The model under review builds one solid part; all positions refer to its coordinate system, in mm. A direction names the side the tool comes from. Coordinates: 2 decimals unless noted, no trailing zeros. Loops run counter-clockwise (first coordinate to the right, second up) from the corner with the lowest first, then second, coordinate; pieces in that order, holes last. Notation, with made-up numbers: (15.25, 17) - (56.25, 17) arc R19 ccw to (56.25, 52) - close; hole circle Ø11 at (1, 8). An arc over 180 degrees is marked (long way). One line per item, written item: value. Start each with the question number.
1. For faces 1 (the face through (7, -1.83, 10)), 2 (the face through (3, 4.99, -5)), list the 3-axis set-ups (+Z, -Z, +X, -X, +Y, -Y) from which the entire face can be reached by the end or side of a thin tool; tool diameter is ignored.
2. We need section A-A, the plane z = 0. Give the boundary of the cut face in (x, y).
3. Mouldability with a two-part tool opening along Y and no side actions: class faces 3 (the face through (11.74, 2.78, 2.61)), 4 (the face through (11.797, 1.658, -6.136)), 5 (the face through (-0.2, 6.26, 5.3)) as +Y half, -Y half, draft (parallel to the pull), parting line (faces both ways), or undercut.
4. Insertion check: P1, Ø4, axis at x = 1.5, y = 2, coming from the +Z side; P2, Ø1.5, axis at x = -4, y = 2, coming from the -Z side; P3, Ø14.5, axis at x = 0, z = 0, coming from the -Y side. Each pin has a flat end and moves straight along its axis. Give the tip position at first contact, or say it passes through.
5. We need section C-C, the plane y = 2.75. Give the boundary of the cut face in (x, z), then the cut area to 3 significant figures.
6. We need section B-B, the plane x = 0. Give the boundary of the cut face in (y, z), then the cut area to 3 significant figures.
7. To check wall thickness, follow line 1 (X direction, y = 3.5, z = 0); line 2 (Z direction, x = -2.75, y = 0); line 3 (Y direction, x = 1.5, z = -8.75). State the ranges of each line that lie inside material, in increasing order.
8. We need section D-D, the plane y = -1. Give the boundary of the cut face in (x, z), then the cut area to 3 significant figures.
from build123d import *


with BuildPart() as part:
    # Sketch1 → Revolve1 (revolve)
    with BuildSketch(Plane.XY, mode=Mode.PRIVATE) as revolve1_sk:
        with BuildLine():
            Line((12.0269, 0.508129433), (12.0269, 4.990057463))
            Line((12.0269, 4.990057463), (5.207, 4.990057463))
            Line((5.207, 4.990057463), (5.08, 6.260057463))
            Line((5.08, 6.260057463), (12.2809, 6.260057463))
            ThreePointArc((12.2809, 6.260057463), (12.99932049, 5.962477952), (13.2969, 5.244057463))
            Line((13.2969, 5.244057463), (13.2969, -1.829842537))
            Line((13.2969, -1.829842537), (12.0269, -1.829842537))
            ThreePointArc((12.0269, -1.829842537), (11.330182262, -0.940102098), (11.802382058, 0.086582375))
            ThreePointArc((11.802382058, 0.086582375), (11.967270876, 0.269325), (12.0269, 0.508129433))
        make_face()
    revolve(revolve1_sk.sketch.rotate(Axis((0, 0, 0), (0, 1, 0)), 90), axis=Axis((0, 0, 0), (0, 1, 0)))


solid = part.part
Findings below:
1. face 1: +Z, -Z, +X, -X, -Y
1. face 2: none
2. outline: (-13.3, -1.83) - (-12.03, -1.83) arc R1.09 ccw to (-11.8, 0.09) arc R0.51 cw to (-12.03, 0.51) - (-12.03, 4.99) - (-5.21, 4.99) - (-5.08, 6.26) - (-12.28, 6.26) arc R1.02 ccw to (-13.3, 5.24) - close; (5.08, 6.26) - (5.21, 4.99) - (12.03, 4.99) - (12.03, 0.51) arc R0.51 cw to (11.8, 0.09) arc R1.09 ccw to (12.03, -1.83) - (13.3, -1.83) - (13.3, 5.24) arc R1.02 ccw to (12.28, 6.26) - close
3. face 3: undercut
3. face 4: draft
3. face 5: +Y half
4. P1: z = 13.3
4. P2: z = -12.89
4. P3: y = 4.99
5. outline: circle Ø26.59 at (0, 0); hole circle Ø24.05 at (0, 0)
5. area: 101 mm2
6. outline: (-1.83, -13.3) - (5.24, -13.3) arc R1.02 ccw to (6.26, -12.28) - (6.26, -5.08) - (4.99, -5.21) - (4.99, -12.03) - (0.51, -12.03) arc R0.51 cw to (0.09, -11.8) arc R1.09 ccw to (-1.83, -12.03) - close; (-1.83, 12.03) arc R1.09 ccw to (0.09, 11.8) arc R0.51 cw to (0.51, 12.03) - (4.99, 12.03) - (4.99, 5.21) - (6.26, 5.08) - (6.26, 12.28) arc R1.02 ccw to (5.24, 13.3) - (-1.83, 13.3) - close
6. area: 39.7 mm2
7. line 1: -13.3 to -12.03, 12.03 to 13.3
7. line 2: -13.01 to -11.36, 11.36 to 13.01
7. line 3: 4.99 to 6.26
8. outline: circle Ø26.59 at (0, 0); hole circle Ø22.68 at (0, 0)
8. area: 152 mm2
